Check sheet for the modelled part. Datum: model origin and axes. Units: mm. Face numbers are marked on the shaded views. Round coordinates to 2 decimals unless told otherwise and drop trailing zeros. Loops run counter-clockwise (first coordinate to the right, second up) from the corner with the lowest first, then second, coordinate; pieces in that order, holes last. Notation, with made-up numbers: (35.25, 64.5) - (72.25, 64.5) arc R4 ccw to (72.25, 70.5) - close; hole circle Ø9 at (-21.75, -33). An arc over 180 degrees is marked (long way). Put each result on its own line as item: value.
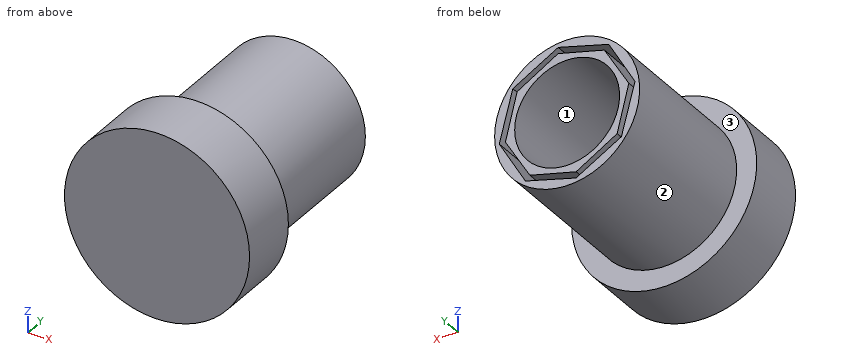
```python
from build123d import *

# Parameters (mm, degrees)
SKETCH1_R           = 17
BOSS_EXTRUDE2_DEPTH = 50
SKETCH3_R           = 23.5
BOSS_EXTRUDE4_DEPTH = 50
SKETCH8_R           = 30
BOSS_EXTRUDE5_DEPTH = 20


with BuildPart() as part:
    # Sketch1 → Boss-Extrude2 (new body)
    with BuildSketch(Plane(origin=(0, 0, 0), x_dir=(1, 0, 0), z_dir=(0, 1, 0))):
        Polygon((16.213203436, -12.071067812), (20, 2.928932188), (12.071067812, 16.213203436), (-2.928932188, 20), (-16.213203436, 12.071067812), (-20, -2.928932188), (-12.071067812, -16.213203436), (2.928932188, -20), align=None)
        Circle(SKETCH1_R, mode=Mode.SUBTRACT)
    extrude(amount=BOSS_EXTRUDE2_DEPTH)



with BuildPart() as body_2:
    # Sketch3 → Boss-Extrude4 (new body)
    with BuildSketch(Plane(origin=(0, 0, 0), x_dir=(1, 0, 0), z_dir=(0, 1, 0))):
        Circle(SKETCH3_R)
        Polygon((-2.890242347, 22), (-17.600059149, 13.512639223), (-22, -2.890242347), (-13.512639223, -17.600059149), (2.890242347, -22), (17.600059149, -13.512639223), (22, 2.890242347), (13.512639223, 17.600059149), align=None, mode=Mode.SUBTRACT)
    extrude(amount=BOSS_EXTRUDE4_DEPTH)


with BuildPart() as part_1:
    add(part.part)

    add(body_2.part)  # Boss-Extrude5 merges body 2
    # Sketch8 → Boss-Extrude5 (add)
    with BuildSketch(Plane(origin=(0, 0, 0), x_dir=(1, 0, 0), z_dir=(0, 1, 0))):
        Circle(SKETCH8_R)
    extrude(amount=-BOSS_EXTRUDE5_DEPTH)


solid = part_1.part
```
Item 1: Release check for a two-part mould opening along Z. For the marked faces 1, 2 and 3 record: +Z half, -Z half, draft (parallel to the pull), parting line (faces both ways), or undercut.
Filled sheet:
face 1: undercut
face 2: parting line
face 3: draft
Item 2: Section check A-A on y = 25. Enter the section's corners in (x, z).
Filled sheet:
outline: circle Ø47 at (0, 0); (-20, 2.93) - (-16.21, -12.07) - (-2.93, -20) - (12.07, -16.21) - (20, -2.93) - (16.21, 12.07) - (2.93, 20) - (-12.07, 16.21) - close; hole (-22, 2.89) - (-17.6, -13.51) - (-2.89, -22) - (13.51, -17.6) - (22, -2.89) - (17.6, 13.51) - (2.89, 22) - (-13.51, 17.6) - close; hole circle Ø34 at (0, 0)
Item 3: Thickness scan on line 1 (X direction, y = 22, z = 0); line 2 (Z direction, x = 2, y = 39). Record the ranges inside material, lowest first. Write a range as from..to.
Filled sheet:
line 1: -23.5..-21.22, -19.26..-17, 17..19.26, 21.22..23.5
line 2: -23.41..-20.69, -18.76..-16.88, 16.88..19.77, 21.76..23.41
Item 4: Section check C-C on z = 2. Enter the section's corners in (x, y), then the cut area to 3 significant figures.
Filled sheet:
outline: (-29.93, -20) - (29.93, -20) - (29.93, 0) - (23.41, 0) - (23.41, 50) - (20.69, 50) - (20.69, 0) - (18.76, 0) - (18.76, 50) - (16.88, 50) - (16.88, 0) - (-16.88, 0) - (-16.88, 50) - (-19.77, 50) - (-19.77, 0) - (-21.76, 0) - (-21.76, 50) - (-23.41, 50) - (-23.41, 0) - (-29.93, 0) - close
area: 1,650 mm²
Item 5: Section check D-D on y = -7. Enter the section's corners in (x, z).
Filled sheet:
outline: circle Ø60 at (0, 0)
Item 6: Section check B-B on x = 10. Enter the section's corners in (y, z), then the cut area to 3 significant figures.
Filled sheet:
outline: (-20, -28.28) - (0, -28.28) - (0, -21.27) - (50, -21.27) - (50, -18.54) - (0, -18.54) - (0, -16.74) - (50, -16.74) - (50, -13.75) - (0, -13.75) - (0, 13.75) - (50, 13.75) - (50, 15.78) - (0, 15.78) - (0, 17.9) - (50, 17.9) - (50, 21.27) - (0, 21.27) - (0, 28.28) - (-20, 28.28) - close
area: 1,690 mm²
Item 7: Go/stop test with flat-tipped pins: pin 1 (10 mm diameter, centred on x = -22, y = 33, fed in from +Z) (3 decimals); pin 2 (8 mm diameter, centred on x = -9.5, y = -1, fed in from -Z); pin 3 (8 mm diameter, centred on y = 16.5, z = -11.5, fed in from +X). Record where each tip stops, or that it passes through.
Filled sheet:
pin 1: z = 16.225
pin 2: z = -29.49
pin 3: x = 22.27
